Read the model definition and answer for the solid it produces. Units are mm, in the model's axes. Face numbers are marked on the shaded views. Coordinates: 2 decimals unless noted, no trailing zeros. Order: outer loops, then holes, each group sorted by start corner. A loop starts at its lowest first (then second) coordinate and runs counter-clockwise, first axis right, second up. Notation, with made-up numbers: (37.5, 58) - (73.5, 58) arc R11 ccw to (73.5, 76) - close; hole circle Ø3 at (-16.75, 4). An arc over 180 degrees is marked (long way). Write item = value, one per line.
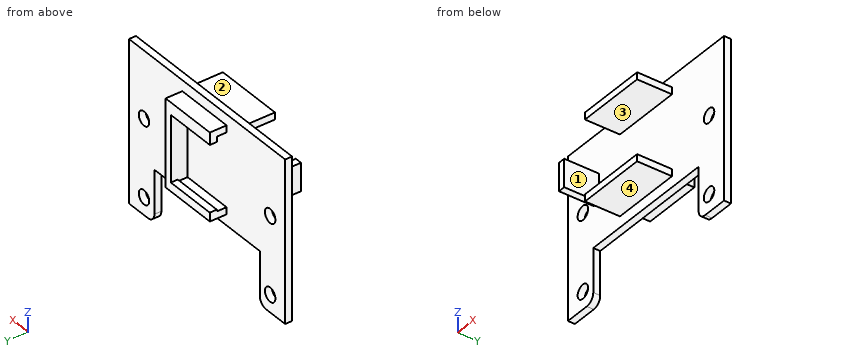
from build123d import *

# Parameters (mm, degrees)
SKETCH1_R           = 2.5527
BOSS_EXTRUDE1_DEPTH = 2.54
SKETCH7_W           = 76.2
SKETCH7_H           = 17.915396906
BOSS_EXTRUDE5_DEPTH = 2.54
BOSS_EXTRUDE2_DEPTH = 3.556
SKETCH4_W           = 31.75
SKETCH4_H           = 3.556
CUT_EXTRUDE1_DEPTH  = 2.54
BOSS_EXTRUDE3_DEPTH = 2.54
BOSS_EXTRUDE4_DEPTH = 12.7


with BuildPart() as part:
    # Sketch1 → Boss-Extrude1 (new body)
    with BuildSketch(Plane(origin=(0, 0, 0), x_dir=(1, 0, 0), z_dir=(0, 1, 0))):
        with BuildLine():
            Line((38.1, -20.3835), (-38.1, -20.3835))
            Line((-38.1, -20.3835), (-38.1, 20.3835))
            Line((-38.1, 20.3835), (-28.8925, 20.3835))
            ThreePointArc((-28.8925, 20.3835), (-26.64743597, 19.45356403), (-25.7175, 17.2085))
            Line((-25.7175, 17.2085), (-25.7175, 1.3335))
            Line((-25.7175, 1.3335), (25.7175, 1.3335))
            Line((25.7175, 1.3335), (25.7175, 17.2085))
            ThreePointArc((25.7175, 17.2085), (26.64743597, 19.45356403), (28.8925, 20.3835))
            Line((28.8925, 20.3835), (38.1, 20.3835))
            Line((38.1, 20.3835), (38.1, -20.3835))
        make_face()
        with Locations(Location((30.7975, -14.0335, 0), (0, 0, 270))):
            Circle(SKETCH1_R, mode=Mode.SUBTRACT)
        with Locations(Location((30.7975, 14.0335, 0), (0, 0, 270))):
            Circle(SKETCH1_R, mode=Mode.SUBTRACT)
        with Locations(Location((-30.7975, -14.0335, 0), (0, 0, 90))):
            Circle(SKETCH1_R, mode=Mode.SUBTRACT)
        with Locations(Location((-30.7975, 14.0335, 0), (0, 0, 90))):
            Circle(SKETCH1_R, mode=Mode.SUBTRACT)
    extrude(amount=BOSS_EXTRUDE1_DEPTH)

    # Sketch7 → Boss-Extrude5 (add)
    with BuildSketch(Plane(origin=(0, 2.54, 0), x_dir=(1, 0, 0), z_dir=(0, 1, 0))):
        with Locations((0, -29.341198453)):
            Rectangle(SKETCH7_W, SKETCH7_H)
    extrude(amount=-BOSS_EXTRUDE5_DEPTH)

    # Sketch3 → Boss-Extrude2 (add)
    with BuildSketch(Plane(origin=(0, 2.54, 0), x_dir=(1, 0, 0), z_dir=(0, 1, 0))):
        Polygon((-12.065, -2.607698453), (-12.065, -5.147698453), (-9.525, -5.147698453), (9.525, -5.147698453), (9.525, -31.817698453), (-9.525, -31.817698453), (-12.065, -31.817698453), (-12.065, -34.357698453), (12.065, -34.357698453), (12.065, -2.607698453), align=None)
    extrude(amount=BOSS_EXTRUDE2_DEPTH)

    # Sketch4 → Cut-Extrude1 (cut)
    with BuildSketch(Plane.ZY.offset(12.065)):
        with Locations((18.482698453, 4.318)):
            Rectangle(SKETCH4_W, SKETCH4_H)
    extrude(amount=-CUT_EXTRUDE1_DEPTH, mode=Mode.SUBTRACT)

    # Sketch5 → Boss-Extrude3 (add)
    with BuildSketch(Plane(origin=(0, 6.096, 0), x_dir=(1, 0, 0), z_dir=(0, 1, 0))):
        Polygon((-9.525, -2.607698453), (-9.525, -5.782698453), (9.525, -5.782698453), (9.525, -29.912698453), (-9.525, -29.912698453), (-9.525, -34.357698453), (12.065, -34.357698453), (12.065, -2.607698453), align=None)
    extrude(amount=BOSS_EXTRUDE3_DEPTH)

    # Sketch6 → Boss-Extrude4 (add)
    with BuildSketch(Plane(origin=(0, 0, 0), x_dir=(-1, 0, 0), z_dir=(0, -1, 0))):
        Polygon((22.86, -13.402698453), (22.86, -18.482698453), (22.86, -23.562698453), (25.4, -23.562698453), (25.4, -13.402698453), align=None)
        Polygon((-12.7, -2.607698453), (-12.7, -5.147698453), (0, -5.147698453), (12.7, -5.147698453), (12.7, -2.607698453), align=None)
        Polygon((-12.7, -31.817698453), (0, -31.817698453), (12.7, -31.817698453), (12.7, -34.357698453), (-12.7, -34.357698453), align=None)
    extrude(amount=BOSS_EXTRUDE4_DEPTH)


solid = part.part
1) Determine the mould class of the marked faces 1, 2, 3 and 4 for opening direction Z: pulls with the +Z half, pulls with the -Z half, needs draft (parallel to the pull), parting line crosses it, or undercut.
Returned:
face_1 = needs draft
face_2 = pulls with the +Z half
face_3 = undercut
face_4 = pulls with the -Z half
2) The part is cut by section C-C (y = 7). Determine the outline of the cut face in (x, z) (3 decimals).
Returned:
outline = (-9.525, 2.608) - (12.065, 2.608) - (12.065, 34.358) - (-9.525, 34.358) - (-9.525, 29.913) - (9.525, 29.913) - (9.525, 5.783) - (-9.525, 5.783) - close
3) Flat-ended cylindrical pins translate along their axes: pin 1 Ø1.5 at (x, y) = (3, -1) entering from +Z; pin 2 Ø10 at (x, y) = (-18, -7) entering from -Z; pin 3 Ø6 at (x, z) = (-10.5, -1) entering from -Y. Find the tip coordinate at first contact, or state that the pin passes through.
Returned:
pin_1 = 34.36
pin_2 = 13.4
pin_3 = 0
4) The part is cut by section A-A (z = -7.5). Determine the outline of the cut face in (x, y).
Returned:
outline = (-38.1, 0) - (-25.72, 0) - (-25.72, 2.54) - (-38.1, 2.54) - close; (25.72, 0) - (38.1, 0) - (38.1, 2.54) - (25.72, 2.54) - close
5) The part is cut by section B-B (y = -3.5). Determine the outline of the cut face in (x, z), and give its area (3 significant figures).
Returned:
outline = (-25.4, 13.4) - (-22.86, 13.4) - (-22.86, 23.56) - (-25.4, 23.56) - close; (-12.7, 2.61) - (12.7, 2.61) - (12.7, 5.15) - (-12.7, 5.15) - close; (-12.7, 31.82) - (12.7, 31.82) - (12.7, 34.36) - (-12.7, 34.36) - close
area = 155 mm^2
6) The part is cut by section D-D (z = 15.5). Determine the outline of the cut face in (x, y) (3 decimals).
Returned:
outline = (-38.1, 0) - (-32.887, 0) - (-32.887, 2.54) - (-38.1, 2.54) - close; (-28.708, 0) - (-25.4, 0) - (-25.4, -12.7) - (-22.86, -12.7) - (-22.86, 0) - (28.708, 0) - (28.708, 2.54) - (12.065, 2.54) - (12.065, 8.636) - (9.525, 8.636) - (9.525, 2.54) - (-28.708, 2.54) - close; (32.887, 0) - (38.1, 0) - (38.1, 2.54) - (32.887, 2.54) - close
7) Straight lines are drawn through the part: line 1 along Z through (x, y) = (-9, -2); line 2 along X through (y, z) = (2.5, -14.5); line 3 along X through (y, z) = (-9, 18). For each, find the intervals that lie inside material, in ascending order. Write a range as from..to.
Returned:
line_1 = 2.61..5.15, 31.82..34.36
line_2 = -38.1..-33.31, -28.29..-25.72, 25.72..28.29, 33.31..38.1
line_3 = -25.4..-22.86
